```python
from build123d import *

# Parameters (mm, degrees)
ESBO_O1_R                = 10.25
RESSALTO_EXTRUS_O1_DEPTH = 3
ESBO_O2_R                = 9.8
CORTE_EXTRUS_O1_DEPTH    = 2.2
ESBO_O3_R                = 6.75
CORTE_EXTRUS_O2_DEPTH    = 15.66168476


with BuildPart() as part:
    # Esboço1 → Ressalto-extrusão1 (new body)
    with BuildSketch(Plane.XY):
        Circle(ESBO_O1_R)
    extrude(amount=RESSALTO_EXTRUS_O1_DEPTH)

    # Esboço2 → Corte-extrusão1 (cut)
    with BuildSketch(Plane(origin=(0, 0, 0), x_dir=(-1, 0, 0), z_dir=(0, 0, -1))):
        Circle(ESBO_O2_R)
    extrude(amount=-CORTE_EXTRUS_O1_DEPTH, mode=Mode.SUBTRACT)

    # Esboço3 → Corte-extrusão2 (cut, through all)
    with BuildSketch(Plane(origin=(0, 0, 2.2), x_dir=(-1, 0, 0), z_dir=(0, 0, -1))):
        Circle(ESBO_O3_R)
    extrude(amount=-CORTE_EXTRUS_O2_DEPTH, mode=Mode.SUBTRACT)


solid = part.part
```
Part model, mm, in its own coordinate system. A direction names the side the tool comes from. Give positions to 0.01 mm unless a question says otherwise; leave off trailing zeros. Order: outer loops, then holes, each group sorted by start corner. A loop starts at its lowest first (then second) coordinate and runs counter-clockwise, first axis right, second up. Notation, with made-up numbers: M -22,30.5 L 35,30.5 A24 ccw 35,45.5 Z; hole C -9.5,21 d8. An arc over 180 degrees is marked long. Use a Markdown table: item, result. Add a question column.
(1) Saw through at A-A, the plane y = 0. Give the cut face in (x, z).
(2) Mould opens along X. For faces 3 (the face through (1.46, -6.59, 2.59)), 4 (the face through (1, -10, 0)), 5 (the face through (-2.222, -10.006, 1.479)) say: +X half, -X half, draft (parallel to the pull), parting line (faces both ways), or undercut.
(3) 3-axis set-ups, long thin cutter, end or side, ignore diameter. For faces 1 (the face through (7, -2, 3)), 2 (the face through (2.124, -9.567, 1.085)): which of +Z, -Z, +X, -X, +Y, -Y reach the whole face in a straight line?
(4) Saw through at D-D, the plane z = 1.35. Give the cut face in (x, y), and give its area (3 significant figures).
(5) Drop flat-ended pins along their axis: P1, Ø1.5, axis at y = -7, z = 1.5, coming from the -X side; P2, Ø12, axis at x = 0, y = 0, coming from the +Z side. Give the stop position or say it passes through.
(6) Probe line 1 along Y through (x, z) = (0, 1.4); line 2 along Z through (x, y) = (7.75, 2.5); line 3 along Y through (x, z) = (0, 2.5). List the from-to ranges inside material, lowest first. Write a range as [from, to].
(7) Saw through at C-C, the plane y = -8.75. Give the cut face in (x, z).
Answer key:
| question | item | result |
|---|---|---|
| 1 | outline | M -10.25,0 L -9.8,0 L -9.8,2.2 L -6.75,2.2 L -6.75,3 L -10.25,3 Z; M 6.75,2.2 L 9.8,2.2 L 9.8,0 L 10.25,0 L 10.25,3 L 6.75,3 Z |
| 2 | face 3 | undercut |
| 2 | face 4 | draft |
| 2 | face 5 | parting line |
| 3 | face 1 | +Z, +X, -X, +Y, -Y |
| 3 | face 2 | -Z |
| 4 | outline | C 0,0 d20.5; hole C 0,0 d19.6 |
| 4 | area | 28.3 mm^2 |
| 5 | P1 | x = -8.12 |
| 5 | P2 | through |
| 6 | line 1 | [-10.25, -9.8], [9.8, 10.25] |
| 6 | line 2 | [2.2, 3] |
| 6 | line 3 | [-10.25, -6.75], [6.75, 10.25] |
| 7 | outline | M -5.34,0 L -4.41,0 L -4.41,2.2 L 4.41,2.2 L 4.41,0 L 5.34,0 L 5.34,3 L -5.34,3 Z |
